from build123d import *

# Parameters (mm, degrees)
SKETCH3_R          = 0.7
CUT_EXTRUDE1_DEPTH = 2


with BuildPart() as part:
    # Sketch2 → Revolve1 (revolve)
    with BuildSketch(Plane(origin=(0, 0, 0), x_dir=(1, 0, 0), z_dir=(0, 1, 0))):
        Polygon((-2.345452762, 2.067742112), (-2.345452762, 3), (-1.845452762, 3), (-0.089526495, 7), (6.910473505, 7), (6.910473505, 5.285375335), (7.110473505, 5.285375335), (7.110473505, 7), (9.954547238, 5.285375335), (9.954547238, 1.223141528), (11.954547238, 1.223141528), (11.954547238, 0), (-8.345452762, 0), (-8.345452762, 2), (-3.845452762, 2), (-3.845452762, 2.067742112), align=None)
    revolve(axis=Axis((11.954547238, 0, 0), (-1, 0, 0)))

    # Sketch3 → Cut-Extrude1 (cut)
    with BuildSketch(Plane(origin=(9.954547238, 0, 0), x_dir=(0, 0, -1), z_dir=(1, 0, 0))):
        with Locations((2.969848481, 2.969848481)):
            Circle(SKETCH3_R)
        with Locations((2.969848481, -2.969848481)):
            Circle(SKETCH3_R)
        with Locations((-2.969848481, -2.969848481)):
            Circle(SKETCH3_R)
        with Locations((-2.969848481, 2.969848481)):
            Circle(SKETCH3_R)
    extrude(amount=-CUT_EXTRUDE1_DEPTH, mode=Mode.SUBTRACT)


solid = part.part
Model file for the job. Use its own axes, mm. A direction names the side the tool comes from. Give positions to 0.01 mm unless a question says otherwise; leave off trailing zeros. Loops run counter-clockwise (first coordinate to the right, second up) from the corner with the lowest first, then second, coordinate; pieces in that order, holes last.
1) Pull direction Y, two halves, no side cores. Call faces 4 (the cylindrical face through (8.969, -3.238, -3.616)), 5 (the cylindrical face through (8.969, -3.238, 2.323)), 6 (the cylindrical face through (3.459, 2.681, -6.466)), 7 (the flat face through (9.955, 1, -1)): +Y half, -Y half, draft (parallel to the pull), parting line (faces both ways), or undercut.
2) Saw through at A-A (z = 0). Write the cut outline in (x, y), plus the area to 3 significant figures.
3) Wall check: line 1 (Z direction, x = 9.5, y = 3.5); line 2 (X direction, y = -1.75, z = 6); line 3 (X direction, y = 1.25, z = -2.25). Give the ranges that are in metal, low to high.
4) Tool access for faces 1 (the flat face through (7.11, -5, 3)), 2 (the cylindrical face through (8.969, 3.664, -2.879)), 3 (the cylindrical face through (-2, 0, 3)): list every direction of +Z, -Z, +X, -X, +Y, -Y with a clear straight run to the whole face (end or side of a thin tool).
5) Flat gauge pins, fed straight in: pin 1 Ø1 at (y, z) = (1.5, -4.5) entering from +X; pin 2 Ø0.8 at (y, z) = (-2.97, -2.97) entering from -X; pin 3 Ø1.1 at (y, z) = (-3, -3) entering from +X; pin 4 Ø3 at (x, y) = (-5, 4.5) entering from -Z. Where does each tip first touch, or does it go through?
Answer block:
1. face 4: undercut
1. face 5: undercut
1. face 6: parting line
1. face 7: draft
2. outline: (-8.35, -2) - (-3.85, -2) - (-3.85, -2.07) - (-2.35, -2.07) - (-2.35, -3) - (-1.85, -3) - (-0.09, -7) - (6.91, -7) - (6.91, -5.29) - (7.11, -5.29) - (7.11, -7) - (9.95, -5.29) - (9.95, -1.22) - (11.95, -1.22) - (11.95, 1.22) - (9.95, 1.22) - (9.95, 5.29) - (7.11, 7) - (7.11, 5.29) - (6.91, 5.29) - (6.91, 7) - (-0.09, 7) - (-1.85, 3) - (-2.35, 3) - (-2.35, 2.07) - (-3.85, 2.07) - (-3.85, 2) - (-8.35, 2) - close
2. area: 185 mm2
3. line 1: z = -4.32 to -3.43, -2.51 to 2.51, 3.43 to 4.32
3. line 2: x = -0.42 to 6.91, 7.11 to 8.35
3. line 3: x = -2.35 to 9.95
4. face 1: none
4. face 2: +X
4. face 3: -X
5. pin 1: stops at x = 9.95
5. pin 2: stops at x = -1.49
5. pin 3: stops at x = 7.95
5. pin 4: passes through
